Input: part model. Units: mm. Frame: model coordinates. A direction names the side the tool comes from. Round coordinates to 2 decimals unless told otherwise and drop trailing zeros. Order: outer loops, then holes, each group sorted by start corner. A loop starts at its lowest first (then second) coordinate and runs counter-clockwise, first axis right, second up. Notation, with made-up numbers: (-7.5, 18) - (21.5, 18) arc R14 ccw to (21.5, 32) - close; hole circle Ø6 at (16, -29). An arc over 180 degrees is marked (long way). One line per item, written item: value. Start each with the question number.
from build123d import *

# Parameters (mm, degrees)
F0_W      = 812.8
F0_H      = 812.8
F0_R      = 55
F0_R_2    = 82.5
F1_DEPTH  = 100
F2_R      = 87.5
F2_R_2    = 55
F3_DEPTH  = 230
F4_W      = 40
F4_H      = 250
F5_DEPTH  = 275
F7_DEPTH  = 362.8
F8_R      = 75
F9_R      = 37.5
F10_DEPTH = 362.8


with BuildPart() as f1:
    # F0 (on Front) → F1 (new body)
    with BuildSketch(Plane.XZ):
        Rectangle(F0_W, F0_H)
        with Locations((-271.4, -271.4)):
            Circle(F0_R, mode=Mode.SUBTRACT)
        Circle(F0_R_2, mode=Mode.SUBTRACT)
        with Locations((271.4, -271.4)):
            Circle(F0_R, mode=Mode.SUBTRACT)
        with Locations((-271.4, 271.4)):
            Circle(F0_R, mode=Mode.SUBTRACT)
        with Locations((271.4, 271.4)):
            Circle(F0_R, mode=Mode.SUBTRACT)
    extrude(amount=F1_DEPTH)

    # F2 (on face) → F3 (join)
    with BuildSketch(Plane.XZ.offset(100)):
        with Locations((-271.4, 271.4)):
            Circle(F2_R)
        with Locations((-271.4, 271.4)):
            Circle(F2_R_2, mode=Mode.SUBTRACT)
        with Locations((271.4, 271.4)):
            Circle(F2_R)
        with Locations((271.4, 271.4)):
            Circle(F2_R_2, mode=Mode.SUBTRACT)
        with Locations((271.4, -271.4)):
            Circle(F2_R)
        with Locations((271.4, -271.4)):
            Circle(F2_R_2, mode=Mode.SUBTRACT)
        with Locations((-271.4, -271.4)):
            Circle(F2_R)
        with Locations((-271.4, -271.4)):
            Circle(F2_R_2, mode=Mode.SUBTRACT)
    extrude(amount=F3_DEPTH)

    # F4 (on face) → F5 (join)
    with BuildSketch(Plane.XZ.offset(100)):
        with Locations((-53.8, 276.4)):
            Rectangle(F4_W, F4_H)
        with Locations((53.8, 276.4)):
            Rectangle(F4_W, F4_H)
        with Locations((161.4, 276.4)):
            Rectangle(F4_W, F4_H)
        with Locations((161.4, -276.4)):
            Rectangle(F4_W, F4_H)
        with Locations((53.8, -276.4)):
            Rectangle(F4_W, F4_H)
        with Locations((-53.8, -276.4)):
            Rectangle(F4_W, F4_H)
        with Locations((-161.4, 276.4)):
            Rectangle(F4_W, F4_H)
        with Locations((-161.4, -276.4)):
            Rectangle(F4_W, F4_H)
    extrude(amount=F5_DEPTH)

    # F6 (on face) → F7 (cut, through all)
    with BuildSketch(Plane(origin=(-181.4, 0, 0), x_dir=(0, -1, 0), z_dir=(-1, 0, 0))):
        Polygon((375, 151.4), (375, 276.4), (100, 151.4), align=None)
        Polygon((375, -151.4), (100, -151.4), (375, -276.4), align=None)
    extrude(amount=-F7_DEPTH, mode=Mode.SUBTRACT)

    # F8
    f8_edges = [f1.edges().sort_by_distance(p)[0] for p in [
        (161.4, -375, 401.4),
        (161.4, -375, 276.4),
        (53.8, -375, 401.4),
        (53.8, -375, 276.4),
        (-53.8, -375, 401.4),
        (-53.8, -375, 276.4),
        (-161.4, -375, 401.4),
        (-161.4, -375, 276.4),
        (-161.4, -375, -276.4),
        (-161.4, -375, -401.4),
        (-53.8, -375, -276.4),
        (-53.8, -375, -401.4),
        (53.8, -375, -276.4),
        (53.8, -375, -401.4),
        (161.4, -375, -276.4),
        (161.4, -375, -401.4),
    ]]
    fillet(f8_edges, radius=F8_R)

    # F9 (on face) → F10 (cut, through all)
    with BuildSketch(Plane(origin=(-181.4, 0, 0), x_dir=(0, -1, 0), z_dir=(-1, 0, 0))):
        with Locations((315, 326.4)):
            Circle(F9_R)
        with Locations((315, -326.4)):
            Circle(F9_R)
    extrude(amount=-F10_DEPTH, mode=Mode.SUBTRACT)


solid = f1.part
Item 1: Section query A-A on z = 0. Return loops of the section in (x, y).
Item 2: First-contact query: pin 1 Ø4 at (x, y) = (199.5, -211) entering from +Z; pin 2 Ø3 at (x, z) = (285, 35.5) entering from -Y; pin 3 Ø4 at (y, z) = (-310, -287.5) entering from -X. Flat tips, straight axial feed; report the tip coordinate or a pass-through.
Item 3: Line query: L1, parallel to Z at x = -267, y = -155; L2, parallel to Z at x = -68, y = -296; L3, parallel to Y at x = -159, z = -326. Output: solid intervals per line, ascending.
Item 4: Reachability of faces 1 (the face through (-33.8, -205, -306)), 2 (the face through (161.12, -287.361, -301.056)), 3 (the face through (-54, -363, 284)) from +Z, -Z, +X, -X, +Y, -Y: full face, straight path, thin tool, end or side. Return the list, or none.
Item 5: Pull-direction query (Y, two-part tool) for faces 4 (the face through (-54, -199, 401.4)), 5 (the face through (161.12, -213.9, -203.173)), 6 (the face through (-54.08, -287.361, -301.056)); classes: released by +Y, released by -Y, zero draft, split by the parting line, or undercut.
Item 6: Section query D-D on y = -247. Give the number of separate pieces and of enclosed holes in the cut face, and give its area (3 significant figures).
Item 7: Section query C-C on y = -80. Return loops of the section in (x, z), and give its area (3 significant figures).
Item 8: Section query B-B on x = 271.4. Return loops of the section in (y, z).
Geometry results:
1. outline: (-406.4, -100) - (-82.5, -100) - (-82.5, 0) - (-406.4, 0) - close; (82.5, -100) - (406.4, -100) - (406.4, 0) - (82.5, 0) - close
2. pin 1: stops at z = 324.03
2. pin 2: stops at y = -100
2. pin 3: stops at x = -357.76
3. L1: z = -358.79 to -326.22, -216.58 to -184.01, 184.01 to 216.58, 326.22 to 358.79
3. L2: z = -401.4 to -358.73, -294.07 to -240.49, 240.49 to 294.07, 358.73 to 401.4
3. L3: y = -375 to -352.5, -277.5 to 0
4. face 1: +Z, -Z, -Y
4. face 2: none
4. face 3: +X, -X, -Y
5. face 4: zero draft
5. face 5: released by -Y
5. face 6: undercut
6. separate pieces: 12
6. enclosed holes: 4
6. area: 117,000 mm^2
7. outline: (-406.4, -406.4) - (406.4, -406.4) - (406.4, 406.4) - (-406.4, 406.4) - close; hole circle Ø110 at (-271.4, -271.4); hole circle Ø110 at (-271.4, 271.4); hole circle Ø165 at (0, 0); hole circle Ø110 at (271.4, -271.4); hole circle Ø110 at (271.4, 271.4)
7. area: 601,000 mm^2
8. outline: (-330, -358.9) - (-100, -358.9) - (-100, -406.4) - (0, -406.4) - (0, -326.4) - (-330, -326.4) - close; (-330, -216.4) - (0, -216.4) - (0, 216.4) - (-330, 216.4) - (-330, 183.9) - (-100, 183.9) - (-100, -183.9) - (-330, -183.9) - close; (-330, 326.4) - (0, 326.4) - (0, 406.4) - (-100, 406.4) - (-100, 358.9) - (-330, 358.9) - close
